Input: part model. Units: mm. Frame: model coordinates. A direction names the side the tool comes from. Give positions to 0.01 mm unless a question says otherwise; leave off trailing zeros. Order: outer loops, then holes, each group sorted by start corner. A loop starts at its lowest first (then second) coordinate and runs counter-clockwise, first axis right, second up. Notation, with made-up numbers: M -36,40 L 11,40 A11 ccw 11,56 Z; hole C -24.75,35.25 d9. An arc over 180 degrees is marked long. Use a Markdown table: item, result.
from build123d import *

# Parameters (mm, degrees)
SKETCH1_R           = 20.25
BOSS_EXTRUDE1_DEPTH = 4


with BuildPart() as part:
    # Sketch1 → Boss-Extrude1 (new body)
    with BuildSketch(Plane.XY):
        with BuildLine():
            Line((10, 0), (190, 0))
            ThreePointArc((190, 0), (197.071067812, 2.928932188), (200, 10))
            Line((200, 10), (200, 50))
            Line((200, 50), (200, 54))
            Line((200, 54), (170, 54))
            Line((170, 54), (170, 50))
            Line((170, 50), (130, 50))
            Line((130, 50), (130, 54))
            Line((130, 54), (70, 54))
            Line((70, 54), (70, 50))
            Line((70, 50), (30, 50))
            Line((30, 50), (30, 54))
            Line((30, 54), (0, 54))
            Line((0, 54), (0, 50))
            Line((0, 50), (0, 10))
            ThreePointArc((0, 10), (2.928932188, 2.928932188), (10, 0))
        make_face()
        with Locations((25, 25)):
            Circle(SKETCH1_R, mode=Mode.SUBTRACT)
        with Locations((75, 25)):
            Circle(SKETCH1_R, mode=Mode.SUBTRACT)
        with Locations((125, 25)):
            Circle(SKETCH1_R, mode=Mode.SUBTRACT)
        with Locations((175, 25)):
            Circle(SKETCH1_R, mode=Mode.SUBTRACT)
    extrude(amount=BOSS_EXTRUDE1_DEPTH)


solid = part.part
1) Cut plane A-A on y = 25. Return loops of the section in (x, z), and give its area (3 significant figures).
Response values:
| item | result |
|---|---|
| outline | M 0,0 L 4.75,0 L 4.75,4 L 0,4 Z; M 45.25,0 L 54.75,0 L 54.75,4 L 45.25,4 Z; M 95.25,0 L 104.75,0 L 104.75,4 L 95.25,4 Z; M 145.25,0 L 154.75,0 L 154.75,4 L 145.25,4 Z; M 195.25,0 L 200,0 L 200,4 L 195.25,4 Z |
| area | 152 mm² |
2) Reachability of faces 4 (the face through (170, 52, 2)), 5 (the face through (100, 54, 2)) from +Z, -Z, +X, -X, +Y, -Y: full face, straight path, thin tool, end or side. Return the list, or none.
Response values:
| item | result |
|---|---|
| face 4 | +Z, -Z, +Y |
| face 5 | +Z, -Z, +X, -X, +Y |
3) First-contact query: pin 1 Ø8 at (x, y) = (162.5, 8.5) entering from -Z. Flat tip, straight axial feed; report the tip coordinate or a pass-through.
Response values:
| item | result |
|---|---|
| pin 1 | stops at z = 0 |
4) Cut plane B-B on x = 20. Return loops of the section in (y, z), and give its area (3 significant figures).
Response values:
| item | result |
|---|---|
| outline | M 0,0 L 5.38,0 L 5.38,4 L 0,4 Z; M 44.62,0 L 54,0 L 54,4 L 44.62,4 Z |
| area | 59.0 mm² |
5) Material intervals for line 1 (Y direction, x = 75, z = 2.15); line 2 (X direction, y = 16, z = 1.6); line 3 (X direction, y = 32, z = 3.1), sorted ascending. Write a range as from..to.
Response values:
| item | result |
|---|---|
| line 1 | y = 0..4.75, 45.25..54 |
| line 2 | x = 0..6.86, 43.14..56.86, 93.14..106.86, 143.14..156.86, 193.14..200 |
| line 3 | x = 0..6, 44..56, 94..106, 144..156, 194..200 |
6) Mould query, pull axis X, two halves, no side actions, for faces 1 (the face through (150, 50, 2)), 2 (the face through (15, 54, 2)), 3 (the face through (200, 32, 2)). Classes: released by +X, released by -X, zero draft, split by the parting line, or undercut.
Response values:
| item | result |
|---|---|
| face 1 | undercut |
| face 2 | zero draft |
| face 3 | released by +X |
7) Cut plane D-D on y = 35. Return loops of the section in (x, z).
Response values:
| item | result |
|---|---|
| outline | M 0,0 L 7.39,0 L 7.39,4 L 0,4 Z; M 42.61,0 L 57.39,0 L 57.39,4 L 42.61,4 Z; M 92.61,0 L 107.39,0 L 107.39,4 L 92.61,4 Z; M 142.61,0 L 157.39,0 L 157.39,4 L 142.61,4 Z; M 192.61,0 L 200,0 L 200,4 L 192.61,4 Z |
8) Cut plane C-C on z = 1.25. Return loops of the section in (x, y), and give its area (3 significant figures).
Response values:
| item | result |
|---|---|
| outline | M 0,10 A10 ccw 10,0 L 190,0 A10 ccw 200,10 L 200,54 L 170,54 L 170,50 L 130,50 L 130,54 L 70,54 L 70,50 L 30,50 L 30,54 L 0,54 Z; hole C 25,25 d40.5; hole C 75,25 d40.5; hole C 125,25 d40.5; hole C 175,25 d40.5 |
| area | 5,280 mm² |
